Geometry check sheet. Reference: the model listing, model coordinates, mm. A direction names the side the tool comes from. Give positions to 0.01 mm unless a question says otherwise; leave off trailing zeros. Order: outer loops, then holes, each group sorted by start corner. A loop starts at its lowest first (then second) coordinate and runs counter-clockwise, first axis right, second up. Notation, with made-up numbers: (62, 12.5) - (69, 12.5) arc R24 cw to (69, 40.5) - close; hole circle Ø3 at (35.5, 0). An arc over 180 degrees is marked (long way). Put each result on its own line as item: value. Start each with the question number.
```python
from build123d import *

# Parameters (mm, degrees)
BOSS_EXTRUDE1_DEPTH      = 25.7
SKETCH2_R                = 15
BOSS_EXTRUDE2_DEPTH      = 1
FILLET1_R                = 1
FILLET2_R                = 2
SKETCH3_R                = 16.5
BOSS_EXTRUDE3_DEPTH      = 42
SKETCH4_R                = 3.175
SKETCH4_R_2              = 1.5
CUT_EXTRUDE1_DEPTH       = 5
BOSS_EXTRUDE4_REACH      = 79.587
BOSS_EXTRUDE4_END_RADIUS = 16.5
SKETCH5_R                = 1.7
SKETCH6_R                = 3.175
SKETCH6_R_2              = 1.5
CUT_EXTRUDE2_DEPTH       = 5


with BuildPart() as part:
    # Sketch1 → Boss-Extrude1 (new body)
    with BuildSketch(Plane.XY):
        with BuildLine():
            Line((-28, 20), (28, 20))
            ThreePointArc((28, 20), (29.414213562, 19.414213562), (30, 18))
            Line((30, 18), (30, -18))
            ThreePointArc((30, -18), (29.414213562, -19.414213562), (28, -20))
            Line((28, -20), (-28, -20))
            ThreePointArc((-28, -20), (-29.414213562, -19.414213562), (-30, -18))
            Line((-30, -18), (-30, 18))
            ThreePointArc((-30, 18), (-29.414213562, 19.414213562), (-28, 20))
        make_face()
    extrude(amount=BOSS_EXTRUDE1_DEPTH)

    # Sketch2 → Boss-Extrude2 (add)
    with BuildSketch(Plane.XY.offset(25.7)):
        Circle(SKETCH2_R)
    extrude(amount=BOSS_EXTRUDE2_DEPTH)

    # Fillet1
    fillet1_edges = [part.edges().sort_by_distance(p)[0] for p in [
        (-15, 0, 25.7),
    ]]
    fillet(fillet1_edges, radius=FILLET1_R - 0.0001)  # a hair under: the kernel refuses the full size

    # Fillet2
    fillet2_edges = [part.edges().sort_by_distance(p)[0] for p in [
        (29.414213562, -19.414213562, 25.7),
        (30, 0, 25.7),
        (29.414213562, 19.414213562, 25.7),
        (0, 20, 25.7),
        (-29.414213562, 19.414213562, 25.7),
        (-30, 0, 25.7),
        (-29.414213562, -19.414213562, 25.7),
        (0, -20, 25.7),
    ]]
    fillet(fillet2_edges, radius=FILLET2_R)

    # Sketch3 → Boss-Extrude3 (add)
    with BuildSketch(Plane.XY.offset(26.7)):
        with Locations(Location((0, 0, 0), (0, 0, 180))):
            Circle(SKETCH3_R)
    extrude(amount=BOSS_EXTRUDE3_DEPTH)

    # Sketch4 → Cut-Extrude1 (cut)
    with BuildSketch(Plane.XZ.offset(20)):
        with Locations(Location((0, 20, 0), (0, 0, 270))):
            Circle(SKETCH4_R)
        with Locations(Location((-8, 20, 0), (0, 0, 270))):
            Circle(SKETCH4_R_2)
        with Locations(Location((8, 20, 0), (0, 0, 90))):
            Circle(SKETCH4_R_2)
    extrude(amount=-CUT_EXTRUDE1_DEPTH, mode=Mode.SUBTRACT)

    # Boss-Extrude4: up to this cylinder (the profile starts inside it)
    boss_extrude4_end = Plane(origin=(0, -6.5, 42), z_dir=(0, 0, -1)) * Cylinder(BOSS_EXTRUDE4_END_RADIUS, 214.174, mode=Mode.PRIVATE)
    # Sketch5 → Boss-Extrude4 (add, up to the surface)
    with BuildSketch(Plane(origin=(0, 0, 0), x_dir=(1, 0, 0), z_dir=(0, 1, 0)), mode=Mode.PRIVATE) as boss_extrude4_sk1:
        with Locations(Location((0, -31.5, 0), (0, 0, 270))):
            Circle(SKETCH5_R)
    boss_extrude4_tool1 = extrude(boss_extrude4_sk1.sketch, amount=-BOSS_EXTRUDE4_REACH, mode=Mode.PRIVATE) & boss_extrude4_end
    add(boss_extrude4_tool1.solids().sort_by_distance((0, 0, 31.5))[0])
    # Sketch5 → Boss-Extrude4 (add, up to the surface)
    with BuildSketch(Plane(origin=(0, 0, 0), x_dir=(1, 0, 0), z_dir=(0, 1, 0)), mode=Mode.PRIVATE) as boss_extrude4_sk2:
        with Locations(Location((0, -39.5, 0), (0, 0, 270))):
            Circle(SKETCH5_R)
    boss_extrude4_tool2 = extrude(boss_extrude4_sk2.sketch, amount=-BOSS_EXTRUDE4_REACH, mode=Mode.PRIVATE) & boss_extrude4_end
    add(boss_extrude4_tool2.solids().sort_by_distance((0, 0, 39.5))[0])
    # Sketch5 → Boss-Extrude4 (add, up to the surface)
    with BuildSketch(Plane(origin=(0, 0, 0), x_dir=(1, 0, 0), z_dir=(0, 1, 0)), mode=Mode.PRIVATE) as boss_extrude4_sk3:
        with Locations(Location((0, -52.5, 0), (0, 0, 270))):
            Circle(SKETCH5_R)
    boss_extrude4_tool3 = extrude(boss_extrude4_sk3.sketch, amount=-BOSS_EXTRUDE4_REACH, mode=Mode.PRIVATE) & boss_extrude4_end
    add(boss_extrude4_tool3.solids().sort_by_distance((0, 0, 52.5))[0])

    # Sketch6 → Cut-Extrude2 (cut)
    with BuildSketch(Plane(origin=(30, 0, 0), x_dir=(0, 0, -1), z_dir=(1, 0, 0))):
        with Locations(Location((-20, 0, 0), (0, 0, 90))):
            Circle(SKETCH6_R)
        with Locations(Location((-20, -8, 0), (0, 0, 90))):
            Circle(SKETCH6_R_2)
        with Locations(Location((-20, 8, 0), (0, 0, 270))):
            Circle(SKETCH6_R_2)
    cut_extrude2 = extrude(amount=-CUT_EXTRUDE2_DEPTH, mode=Mode.SUBTRACT)

    # Mirror1: Cut-Extrude2 across plane
    add(cut_extrude2.mirror(Plane(origin=(0, 0, 0), x_dir=(0, 0, 1), z_dir=(1, 0, 0))), mode=Mode.SUBTRACT)


solid = part.part
```
Item 1: Set-up check for faces 5 (the face through (-4, 15, 26.7)), 6 (the face through (25, 8, 20)), 7 (the face through (0, -15, 20)): record each of +Z, -Z, +X, -X, +Y, -Y from which the full face is reachable in a straight line by a thin tool's end or side.
Item 2: Release check for a two-part mould opening along X. For faces 1 (the face through (-8.9, -17.5, 21.2)), 2 (the face through (-30, 0, 12)), 3 (the face through (0.39, 19.4, 25.13)), 4 (the face through (0, -23, 52)) record: +X half, -X half, draft (parallel to the pull), parting line (faces both ways), or undercut.
Item 3: Thickness scan on line 1 along X through (y, z) = (-16.6, 20) (3 decimals); line 2 along Z through (x, y) = (-27.55, 8); line 3 along Z through (x, y) = (-27, 0) (3 decimals). Record the ranges inside material, lowest first.
Item 4: Cross-section at A-A (x = -18.5). Enter the section's corners in (y, z), and give its area (3 significant figures).
Item 5: Cross-section at C-C (z = 58). Enter the section's corners in (x, y), and give its area (3 significant figures).
Item 6: Gauge pin test, flat ends, axial feed: pin 1 Ø1.5 at (x, z) = (-7.5, 19.5) entering from -Y; pin 2 Ø1 at (y, z) = (10.5, 35.5) entering from -X; pin 3 Ø1.5 at (y, z) = (-8.5, 20) entering from -X. Record the tip position at first contact, or that the pin passes through.
Recorded:
1. face 5: none
1. face 6: +X
1. face 7: -Y
2. face 1: undercut
2. face 2: -X half
2. face 3: draft
2. face 4: parting line
3. line 1: x = -30 to -9.5, -6.5 to -3.175, 3.175 to 6.5, 9.5 to 30
3. line 2: z = 0 to 18.5, 21.5 to 25.7
3. line 3: z = 0 to 16.825, 23.175 to 25.7
4. outline: (-20, 0) - (20, 0) - (20, 23.7) arc R2 ccw to (18, 25.7) - (-18, 25.7) arc R2 ccw to (-20, 23.7) - close
4. area: 1,030 mm^2
5. outline: circle Ø33 at (0, 0)
5. area: 855 mm^2
6. pin 1: stops at y = -15
6. pin 2: stops at x = -13.12
6. pin 3: stops at x = -25
